Job drawing, mm, ordinate dimensions from the low corner. One solid piece. A direction names the side the tool comes from. Coordinates: 2 decimals unless noted, no trailing zeros. Order: outer loops, then holes, each group sorted by start corner. A loop starts at its lowest first (then second) coordinate and runs counter-clockwise, first axis right, second up. Notation, with made-up numbers: (-40, 13) - (12, 13) arc R16 cw to (12, 24) - close; hole circle Ø7 at (-22.5, 52.25). An arc over 180 degrees is marked (long way). Return JSON: item names as keys, results as strings.
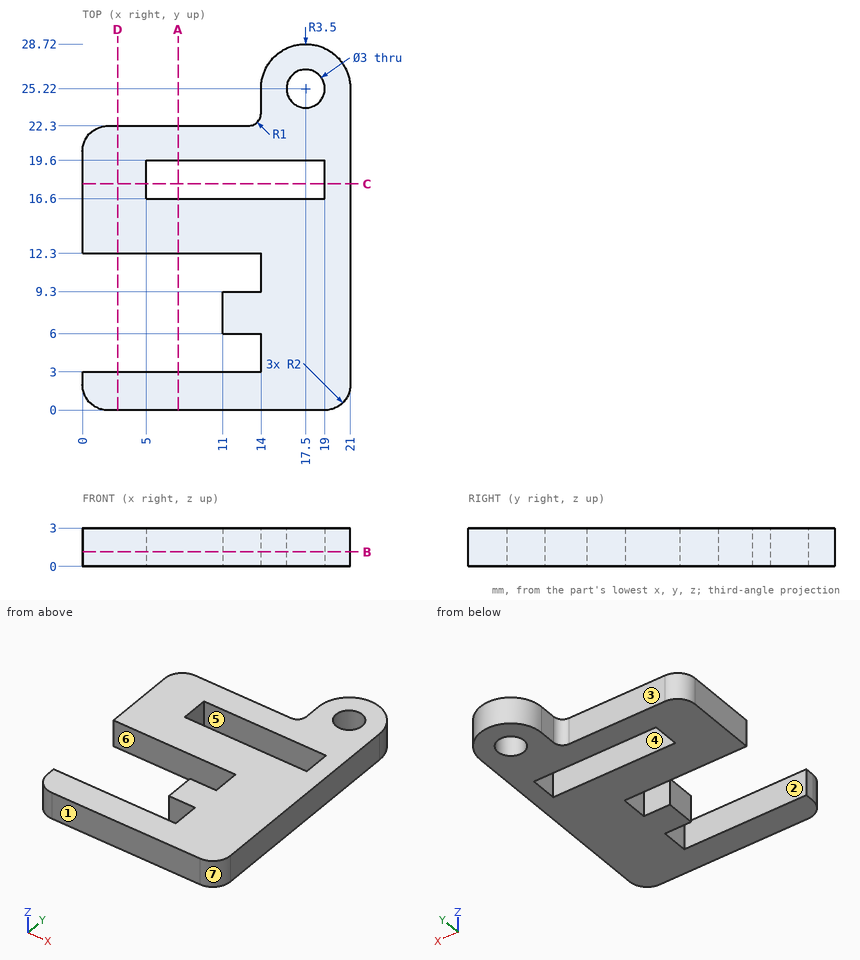
1. Cut at C-C on y = 17.75. Give the cut face in (x, z).
Check values:
{"outline": "(0, 0) - (5, 0) - (5, 3) - (0, 3) - close; (19, 0) - (21, 0) - (21, 3) - (19, 3) - close"}
2. Probe L1, parallel to Y at x = 17.5, z = 2.25; L2, parallel to Y at x = 6.25, z = 0.7; L3, parallel to Y at x = 2.5, z = 0.45. List the from-to ranges inside material, lowest first.
Check values:
{"L1": "0 to 16.6, 19.6 to 23.72, 26.72 to 28.72", "L2": "0 to 3, 12.3 to 16.6, 19.6 to 22.3", "L3": "0 to 3, 12.3 to 22.3"}
3. Tool access for the marked faces 1, 2 and 3: list every direction of +Z, -Z, +X, -X, +Y, -Y with a clear straight run to the whole face (end or side of a thin tool).
Check values:
{"face 1": "+Z, -Z, +X, -X, -Y", "face 2": "+Z, -Z, -X", "face 3": "+Z, -Z, -X, +Y"}
4. Cut at A-A on x = 7.5. Give the cut face in (y, z), plus the area to 3 significant figures.
Check values:
{"outline": "(0, 0) - (3, 0) - (3, 3) - (0, 3) - close; (12.3, 0) - (16.6, 0) - (16.6, 3) - (12.3, 3) - close; (19.6, 0) - (22.3, 0) - (22.3, 3) - (19.6, 3) - close", "area": "30.0 mm²"}
5. Cut at D-D on x = 2.75. Give the cut face in (y, z), plus the area to 3 significant figures.
Check values:
{"outline": "(0, 0) - (3, 0) - (3, 3) - (0, 3) - close; (12.3, 0) - (22.3, 0) - (22.3, 3) - (12.3, 3) - close", "area": "39.0 mm²"}
6. Mould opens along X. For the marked faces 4, 5, 6 and 7 say: pulls with the +X half, pulls with the -X half, needs draft (parallel to the pull), parting line crosses it, or undercut.
Check values:
{"face 4": "undercut", "face 5": "undercut", "face 6": "needs draft", "face 7": "pulls with the +X half"}
7. Drop flat-ended pins along their axis: pin 1 (1.5 mm diameter, centred on y = 4.5, z = 1.5, fed in from -X); pin 2 (1.5 mm diameter, centred on x = 10, z = 1.5, fed in from +Y); pin 3 (1.5 mm diameter, centred on y = 7, z = 1.5, fed in from -X). Give the stop position or say it passes through.
Check values:
{"pin 1": "x = 14", "pin 2": "y = 22.3", "pin 3": "x = 11"}
8. Cut at B-B on z = 1.15. Give the cut face in (x, y), plus the area to 3 significant figures.
Check values:
{"outline": "(0, 2) arc R2 ccw to (2, 0) - (19, 0) arc R2 ccw to (21, 2) - (21, 25.22) arc R3.5 ccw to (14, 25.22) - (14, 23.3) arc R1 cw to (13, 22.3) - (2, 22.3) arc R2 ccw to (0, 20.3) - (0, 12.3) - (14, 12.3) - (14, 9.3) - (11, 9.3) - (11, 6) - (14, 6) - (14, 3) - (0, 3) - close; hole (5, 16.6) - (19, 16.6) - (19, 19.6) - (5, 19.6) - close; hole circle Ø3 at (17.5, 25.22)", "area": "336 mm²"}
